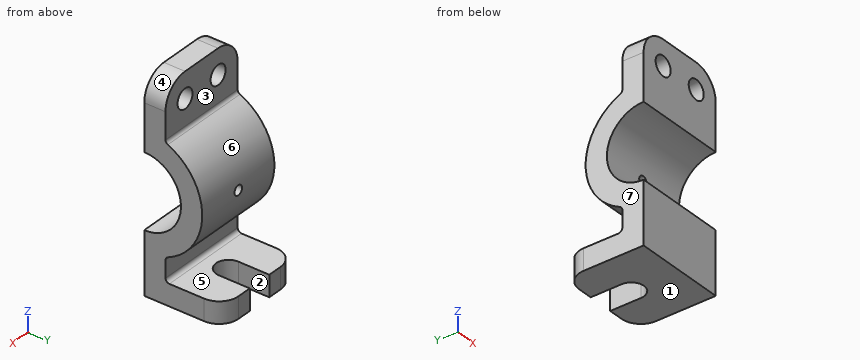
Autodesk Inventor part; units mm, degrees
ref_plane "YZ Plane" through (0, 0, 0) normal (1, 0, 0) x (0, 1, 0)
ref_plane "XZ Plane" through (0, 0, 0) normal (0, 1, 0) x (-1, 0, 0)
ref_plane "XY Plane" through (0, 0, 0) normal (0, 0, 1) x (1, 0, 0)
sketch "Sketch1" plane through (0, 0, 0) normal (1, 0, 0) x (0, 1, 0)
  line L0 (41, 0) -> (0, 0)
  line L1 (0, 0) -> (0, 32)
  arc A0 (0, 32) -> (0, 70) centre (0, 51) ccw
  line L2 (0, 70) -> (0, 107)
  line L3 (41, 11) -> (11, 11)
  line L4 (11, 11) -> (11, 23.0894)
  arc A1 (11, 23.0894) -> (11, 78.9106) centre (0, 51) ccw
  line L5 (11, 78.9106) -> (11, 107)
  line L6 (11, 107) -> (0, 107)
  line L7 (41, 11) -> (41, 0)
  dimension "d0" = 41
  dimension "d1" = 107
  dimension "d2" = 51
  dimension "d3" = 11
  dimension "d4" = 30
extrude "Extrusion1" add sketch "Sketch1" along normal mid plane 48
fillet "Fillet1" radius 13 2 edges at (24, 5.5, 107) (-24, 5.5, 107)
fillet "Fillet2" radius 2 3 edges at (0, 11, 78.9106) (0, 11, 23.0894) (0, 11, 11)
sketch "Sketch2" plane through (-11, 11, 107) normal (0, 1, 0) x (1, 0, 0)
  arc A0 (-13, 13) -> (0, 0) centre (0, 13) ccw
  circle A1 centre (0, 13) radius 5
  circle A2 centre (22, 13.2869) radius 5
  point P0 (11, 107)
  dimension "d9" = 10
  dimension "d10" = 10
extrude "Extrusion2" cut sketch "Sketch2" against normal through all
sketch "Sketch3" plane through (24, 41, 0) normal (0, 0, -1) x (-1, 0, 0)
  line L0 (48, 0) -> (0, 0)
  line L1 (24, 0) -> (24, -16) construction
  line L2 (30.5, 0) -> (17.5, 0)
  line L3 (17.5, 0) -> (17.5, -16)
  line L4 (30.5, -16) -> (30.5, 0)
  arc A0 (17.5, -16) -> (30.5, -16) centre (24, -16) ccw
  point P0 (24, -41)
  dimension "d14" = 13
  dimension "d15" = 6.5
  dimension "d16" = 16
  dimension "d17" = 6.5
extrude "Extrusion3" cut sketch "Sketch3" against normal blind 11
fillet "Fillet3" radius 10 2 edges at (24, 41, 5.5) (-24, 41, 5.5)
sketch "Sketch4" plane through (-24, 0, 0) normal (0, -1, 0) x (1, 0, 0)
  line L0 (48, 70) -> (48, 32)
  line L1 (48, 51) -> (0, 51)
  line L2 (0, 78.4129) -> (0, 23.5871)
  circle A0 centre (24, 51) radius 2.5
  point P0 (24, 0)
  dimension "d21" = 5
extrude "Extrusion4" cut sketch "Sketch4" against normal through all
thread "Thread1"
properties part number "T05"
Model file for the job. Use its own axes, mm. Face numbers are marked on the shaded views. A direction names the side the tool comes from. Give positions to 0.01 mm unless a question says otherwise; leave off trailing zeros. Loops run counter-clockwise (first coordinate to the right, second up) from the corner with the lowest first, then second, coordinate; pieces in that order, holes last. Notation, with made-up numbers: (-10.75, 14.25) - (35.25, 14.25) arc R33 ccw to (35.25, 51.25) - close; hole circle Ø7 at (26, 72.5). An arc over 180 degrees is marked (long way). Use one line per item in the form item = value.
(1) Cut at C-C (x = 0). Give the cut face in (y, z).
Determined:
outline = (0, 0) - (18.5, 0) - (18.5, 11) - (13, 11) arc R2 cw to (11, 13) - (11, 21.76) arc R2 cw to (12.19, 23.59) arc R30 ccw to (29.9, 48.5) - (18.83, 48.5) arc R19 cw to (0, 32) - close; (0, 70) arc R19 cw to (18.83, 53.5) - (29.9, 53.5) arc R30 ccw to (12.19, 78.41) arc R2 cw to (11, 80.24) - (11, 107) - (0, 107) - close
(2) Drill centre lines: L1, parallel to X at y = 8, z = 94; L2, parallel to Z at x = 14.5, y = 13; L3, parallel to Z at x = -6, y = 12. Where is each one in solid material? Low to high.
Determined:
L1 = -24 to -16, -6 to 6.01, 15.99 to 24
L2 = 0 to 11, 23.96 to 37.14, 64.86 to 78.04
L3 = 0 to 11.27, 23.49 to 36.27, 65.73 to 78.51
(3) Cut at A-A (y = 9.5). Give the cut face in (x, z), then the cut area to 3 significant figures.
Determined:
outline = (-24, 0) - (24, 0) - (24, 34.55) - (-24, 34.55) - close; (-24, 67.45) - (24, 67.45) - (24, 94) arc R13 ccw to (11, 107) - (-11, 107) arc R13 ccw to (-24, 94) - close; hole circle Ø10 at (-11, 94); hole circle Ø10 at (11, 93.71)
area = 3,330 mm^2
(4) Pull direction Z, two halves, no side cores. Call the marked faces 4, 5, 6 and 7: pulls with the +Z half, pulls with the -Z half, needs draft (parallel to the pull), parting line crosses it, or undercut.
Determined:
face_4 = pulls with the +Z half
face_5 = undercut
face_6 = undercut
face_7 = needs draft
(5) Cut at B-B (z = 51). Give the cut face in (x, y), then the cut area to 3 significant figures.
Determined:
outline = (-24, 19) - (-2.5, 19) - (-2.5, 30) - (-24, 30) - close; (2.5, 19) - (24, 19) - (24, 30) - (2.5, 30) - close
area = 473 mm^2
(6) Drop flat-ended pins along their axis: P1, Ø2, axis at x = -12, z = 30.5, coming from the +Y side; P2, Ø11.5, axis at x = -11, z = 94, coming from the -Y side; P3, Ø13.5, axis at x = 10, z = 99.5, coming from the +Y side; P4, Ø8, axis at x = 11, z = 93.71, coming from the +Y side. Give the stop position or say it passes through.
Determined:
P1 = 22.8
P2 = 0
P3 = 11
P4 = through
(7) 3-axis set-ups, long thin cutter, end or side, ignore diameter. For the marked faces 1, 2 and 3: which of +Z, -Z, +X, -X, +Y, -Y reach the whole face in a straight line?
Determined:
face_1 = -Z, +X, -X, +Y, -Y
face_2 = -Z, +Y
face_3 = +Z, +X, -X, +Y
(8) Cut at D-D (y = 29). Give the cut face in (x, z), then the cut area to 3 significant figures.
Determined:
outline = (-24, 0) - (-6.5, 0) - (-6.5, 11) - (-24, 11) - close; (-24, 43.32) - (24, 43.32) - (24, 58.68) - (-24, 58.68) - close; (6.5, 0) - (24, 0) - (24, 11) - (6.5, 11) - close; hole circle Ø5 at (0, 51)
area = 1,100 mm^2
